```python
from build123d import *

# Parameters (mm, degrees)
SKETCH1_R           = 10
BOSS_EXTRUDE1_DEPTH = 10
SKETCH2_W           = 5
SKETCH2_H           = 5


with BuildPart() as part:
    # Sketch1 → Boss-Extrude1 (new body)
    with BuildSketch(Plane.XY):
        Circle(SKETCH1_R)
    extrude(amount=BOSS_EXTRUDE1_DEPTH)

    # Sketch2 → Cut-Revolve1 (revolve, cut)
    with BuildSketch(Plane(origin=(0, 0, 0), x_dir=(0, 0, -1), z_dir=(1, 0, 0)), mode=Mode.PRIVATE) as cut_revolve1_sk:
        with Locations((-5, 7.5)):
            Rectangle(SKETCH2_W, SKETCH2_H)
    revolve(cut_revolve1_sk.sketch.rotate(Axis((0, 0, 10), (0, 0, -1)), 90), axis=Axis((0, 0, 10), (0, 0, -1)), mode=Mode.SUBTRACT)


solid = part.part
```
Part model, mm, in its own coordinate system. A direction names the side the tool comes from. Coordinates: 2 decimals unless noted, no trailing zeros. Write each loop counter-clockwise with the first axis right and the second up, starting at its lowest first coordinate (ties: lowest second). Pieces come first, ordered by that corner, then holes.
Item 1: Probe line 1 (Z direction, x = 5.25, y = 2.75); line 2 (Y direction, x = -3.75, z = 0.5); line 3 (Y direction, x = -3.25, z = 1.5). List the from-to ranges inside material, lowest first.
Item 2: Mould opens along Z. For faces 3 (the face through (-2.17, -9.76, 8.73)), 4 (the face through (0, 0, 10)), 5 (the face through (-2, -5, 7.5)) say: released by +Z, released by -Z, zero draft, split by the parting line, or undercut.
Item 3: Slice it at A-A (y = -8). Write the cut outline in (x, z).
Item 4: Slice it at B-B (x = 5.25). Write the cut outline in (y, z), and give its area (3 significant figures).
Item 5: Slice it at C-C (x = 0). Write the cut outline in (y, z).
Item 6: Pin check, flat tip, straight feed: pin 1 (4 mm diameter, centred on x = 0, y = -4, fed in from -Z). Stop position of the tip, or through.
Item 7: Which spindle directions (+Z, -Z, +X, -X, +Y, -Y) get a long thin tool onto all of the face, cutting with end or side? Do faces 1 (the face through (0, 0, 0)), 2 (the face through (-5, 0, 5)). Say none if no direction does.
Results found:
1. line 1: z = 0 to 2.5, 7.5 to 10
1. line 2: y = -9.27 to 9.27
1. line 3: y = -9.46 to 9.46
2. face 3: zero draft
2. face 4: released by +Z
2. face 5: undercut
3. outline: (-6, 0) - (6, 0) - (6, 2.5) - (-6, 2.5) - close; (-6, 7.5) - (6, 7.5) - (6, 10) - (-6, 10) - close
4. outline: (-8.51, 0) - (8.51, 0) - (8.51, 2.5) - (-8.51, 2.5) - close; (-8.51, 7.5) - (8.51, 7.5) - (8.51, 10) - (-8.51, 10) - close
4. area: 85.1 mm2
5. outline: (-10, 0) - (10, 0) - (10, 2.5) - (5, 2.5) - (5, 7.5) - (10, 7.5) - (10, 10) - (-10, 10) - (-10, 7.5) - (-5, 7.5) - (-5, 2.5) - (-10, 2.5) - close
6. pin 1: stops at z = 0
7. face 1: -Z, +X, -X, +Y, -Y
7. face 2: none
